Part model, mm, in its own coordinate system. A direction names the side the tool comes from. Round coordinates to 2 decimals unless told otherwise and drop trailing zeros. Write each loop counter-clockwise with the first axis right and the second up, starting at its lowest first coordinate (ties: lowest second). Pieces come first, ordered by that corner, then holes.
Autodesk Fusion 360 part; units mm, degrees
sketch "Sketch1" plane through (0, 0, 0) normal (0, 0, 1) x (1, 0, 0) in component "Component"
  circle A0 centre (0, 0) radius 3.9687
  dimension "d1" = 7.9375
extrude "Extrude1" add sketch "Sketch1" along normal blind 10 in component "Component"
sketch "Sketch2" plane through (0, 0, 10) normal (0, 0, 1) x (-1, 0, 0) in component "Component"
  circle A0 centre (0, 0) radius 3.9687
  circle A1 centre (0, 0) radius 7.5
  dimension "d4" = 15
extrude "Extrude2" add sketch "Sketch2" along normal blind 2 contours A0 | A1 in component "Component"
sketch "Sketch3" plane through (0, 0, 12) normal (0, 0, 1) x (-1, 0, 0) in component "Component"
  circle A0 centre (0, 0) radius 7.5
  circle A1 centre (0, 0) radius 2.5
  dimension "d7" = 5
extrude "Extrude3" add sketch "Sketch3" along normal blind 24 contours A1 in component "Component"
thread "Thread1" in component "Component"
hole "Hole1" at (0.1045, -0.0914, 0) direction (0, 0, 1) diameter 3 depth 10 tip angle 180 in component "Component"
component "Component" placed x (1, 0, 0) y (0, 1, 0) z (0, 0, 1) at (0, 0, 0)
equation "d1 = ( 5 / 16 ) * 1 in"
Q1. Cut at B-B on x = 1. Write the cut outline in (y, z), plus the area to 3 significant figures.
Values follow:
outline: (-7.43, 10) - (-3.84, 10) - (-3.84, 0) - (-1.29, 0) - (-1.29, 10) - (1.11, 10) - (1.11, 0) - (3.84, 0) - (3.84, 10) - (7.43, 10) - (7.43, 12) - (2.29, 12) - (2.29, 36) - (-2.29, 36) - (-2.29, 12) - (-7.43, 12) - close
area: 192 mm2
Q2. Drop flat-ended pins along their axis: pin 1 (6 mm diameter, centred on x = -4.5, z = 9, fed in from +Y); pin 2 (6 mm diameter, centred on x = -0.5, y = -4, fed in from +Z); pin 3 (8 mm diameter, centred on y = 5, z = 30, fed in from -X); pin 4 (5 mm diameter, centred on y = -1.5, z = 23, fed in from +X). Give the stop position or say it passes through.
Values follow:
pin 1: stops at y = 7.31
pin 2: stops at z = 36
pin 3: stops at x = -2.29
pin 4: stops at x = 2.5
Q3. Which spindle directions (+Z, -Z, +X, -X, +Y, -Y) get a long thin tool onto all of the face, cutting with end or side? Do faces 5 (the flat face through (2, -2, 12)), 6 (the flat face through (-3, 3, 10)), 7 (the cylindrical face through (7.493, 0.33, 10.986)). Say none if no direction does.
Values follow:
face 5: +Z
face 6: -Z
face 7: +Z, -Z
Q4. Cut at D-D on x = -1.75. Write the cut outline in (y, z).
Values follow:
outline: (-7.29, 10) - (-3.56, 10) - (-3.56, 0) - (3.56, 0) - (3.56, 10) - (7.29, 10) - (7.29, 12) - (1.79, 12) - (1.79, 36) - (-1.79, 36) - (-1.79, 12) - (-7.29, 12) - close
Q5. Mould opens along Y. For faces 1 (the flat face through (0, 0, 10)), 2 (the cylindrical face through (1.02, -1.28, 5.07)), 3 (the flat face through (0, 0, 36)), 4 (the cylindrical face through (-0.86, 3.874, 4.93)) say: +Y half, -Y half, draft (parallel to the pull), parting line (faces both ways), or undercut.
Values follow:
face 1: undercut
face 2: undercut
face 3: draft
face 4: parting line
Q6. Cut at C-C on y = -3. Write the cut outline in (x, z), plus the area to 3 significant figures.
Values follow:
outline: (-6.87, 10) - (-2.6, 10) - (-2.6, 0) - (2.6, 0) - (2.6, 10) - (6.87, 10) - (6.87, 12) - (-6.87, 12) - close
area: 79.5 mm2
Q7. Cut at A-A on y = 1. Write the cut outline in (x, z), plus the area to 3 significant figures.
Values follow:
outline: (-7.43, 10) - (-3.84, 10) - (-3.84, 0) - (-0.92, 0) - (-0.92, 10) - (1.13, 10) - (1.13, 0) - (3.84, 0) - (3.84, 10) - (7.43, 10) - (7.43, 12) - (2.29, 12) - (2.29, 36) - (-2.29, 36) - (-2.29, 12) - (-7.43, 12) - close
area: 196 mm2
Q8. Wall check: L1, parallel to Z at x = -1.5, y = -5.25; L2, parallel to Y at x = 0.25, z = 7.5; L3, parallel to X at y = 1, z = 4. Give the ranges that are in metal, low to high.
Values follow:
L1: z = 10 to 12
L2: y = -3.96 to -1.58, 1.4 to 3.96
L3: x = -3.84 to -0.92, 1.13 to 3.84
